Input: dimensioned drawing with shaded views. Units: mm. Origin: part minimum x, y, z. Round coordinates to 2 decimals unless told otherwise and drop trailing zeros. Write each loop counter-clockwise with the first axis right and the second up, starting at its lowest first coordinate (ties: lowest second). Pieces come first, ordered by that corner, then holes. Notation, with made-up numbers: (-8.5, -28) - (20.5, -28) arc R10 ccw to (20.5, -23) - close; hole circle Ø11 at (47.5, 19.5). An arc over 180 degrees is marked (long way). Use one line per item in the form item = value.
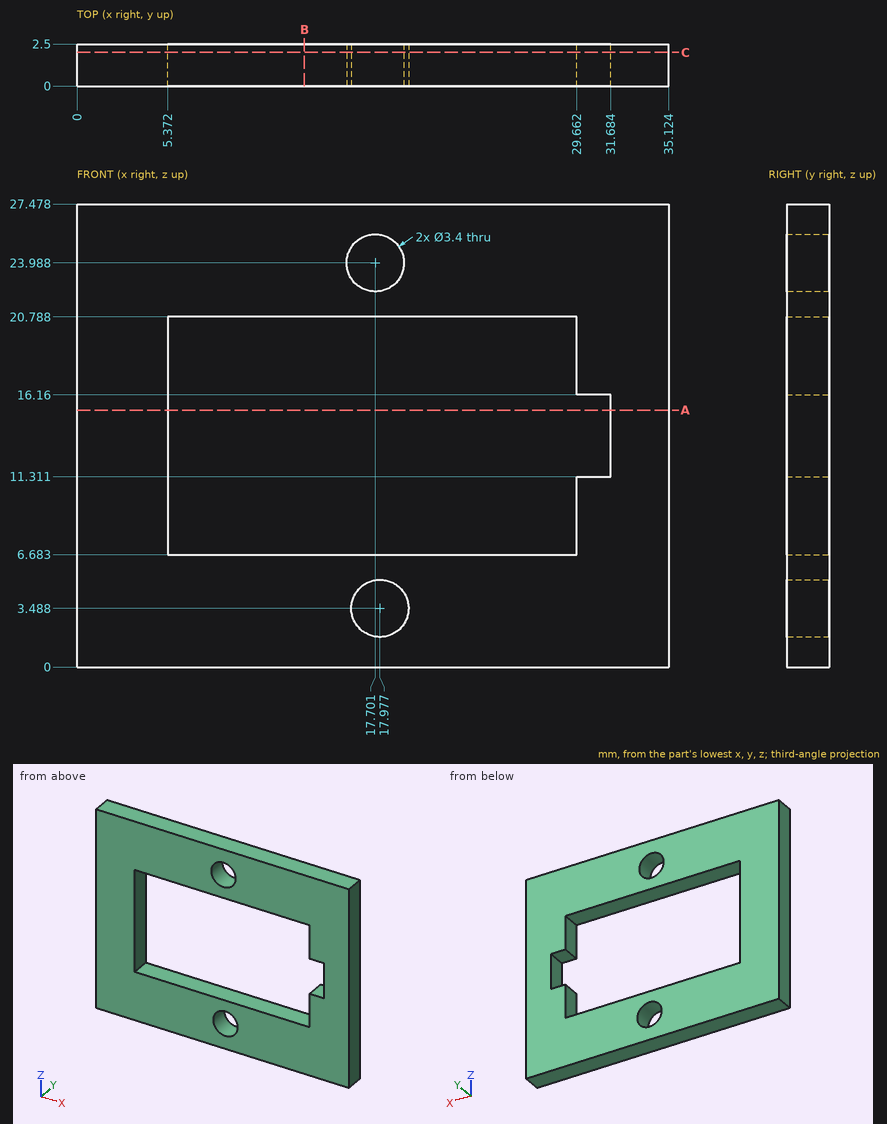
(1) Material intervals for L1, parallel to Z at x = 29.5, y = 1.75; L2, parallel to X at y = 0.85, z = 10.25 (1 decimal); L3, parallel to X at y = 2.1, z = 11.75 (1 decimal), sorted ascending.
Derived:
L1 = 0 to 6.68, 20.79 to 27.48
L2 = 0 to 5.4, 29.7 to 35.1
L3 = 0 to 5.4, 31.7 to 35.1
(2) Cut plane A-A on z = 15.25. Output: boundary loops of the cut face in (x, y) (1 decimal).
Derived:
outline = (0, 0) - (5.4, 0) - (5.4, 2.5) - (0, 2.5) - close; (31.7, 0) - (35.1, 0) - (35.1, 2.5) - (31.7, 2.5) - close
(3) Cut plane B-B on x = 13.5. Output: boundary loops of the cut face in (y, z).
Derived:
outline = (0, 0) - (2.5, 0) - (2.5, 6.68) - (0, 6.68) - close; (0, 20.79) - (2.5, 20.79) - (2.5, 27.48) - (0, 27.48) - close
(4) First-contact query: pin 1 Ø12 at (x, z) = (23, 11) entering from +Y. Flat tip, straight axial feed; report the tip coordinate or a pass-through.
Derived:
pin_1 = 2.5
(5) Cut plane C-C on y = 2. Output: boundary loops of the cut face in (x, z) (1 decimal).
Derived:
outline = (0, 0) - (35.1, 0) - (35.1, 27.5) - (0, 27.5) - close; hole (5.4, 6.7) - (29.7, 6.7) - (29.7, 11.3) - (31.7, 11.3) - (31.7, 16.2) - (29.7, 16.2) - (29.7, 20.8) - (5.4, 20.8) - close; hole circle Ø3.4 at (17.7, 24); hole circle Ø3.4 at (18, 3.5)
